Here's how the part is built. I have some questions about the finished solid (model axes, mm). Face numbers are marked on the shaded views. A direction names the side the tool comes from. Give positions to 0.01 mm unless a question says otherwise; leave off trailing zeros. Write each loop counter-clockwise with the first axis right and the second up, starting at its lowest first coordinate (ties: lowest second). Pieces come first, ordered by that corner, then holes. Notation, with made-up numbers: (-29, 17) -> (-20, 17) arc R17 ccw to (-20, 39) -> close; hole circle Ø3 at (75.25, 16.25). An arc over 180 degrees is marked (long way). Use one line per item in the form item = value.
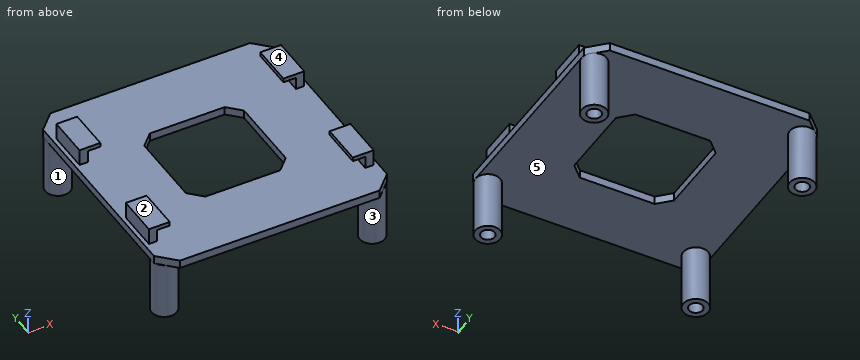
```python
from build123d import *

# Parameters (mm, degrees)
EXTRUDE_START              = -6
EXTRUDE_275_DEPTH          = 2
EXTRUDE_START_2            = -20
SKETCH_2_R                 = 3
EXTRUDE_1_1_DEPTH          = 14
CUT_EXTRUDE_START          = -20
SKETCH_3_R                 = 1.65
CUT_EXTRUDE_M3_1_1_DEPTH   = 14
EXTRUDE_START_3            = -4
SKETCH_4_W                 = 2
SKETCH_4_H                 = 10
EXTRUDE_1_1_2_DEPTH        = 3
EXTRUDE_START_4            = -1
SKETCH_5_W                 = 5
SKETCH_5_H                 = 10
EXTRUDE_1_1_3_DEPTH        = 1
SKETCH_6_R                 = 3
EXTRUDE_1_1_4_DEPTH        = 14
SKETCH_7_R                 = 1.65
CUT_EXTRUDE_M3_1_1_2_DEPTH = 14
SKETCH_8_W                 = 2
SKETCH_8_H                 = 10
EXTRUDE_1_1_5_DEPTH        = 3
SKETCH_9_W                 = 5
SKETCH_9_H                 = 10
EXTRUDE_1_1_6_DEPTH        = 1
SKETCH_10_R                = 3
EXTRUDE_1_1_7_DEPTH        = 14
SKETCH_11_R                = 1.65
CUT_EXTRUDE_M3_1_1_3_DEPTH = 14
SKETCH_12_W                = 2
SKETCH_12_H                = 10
EXTRUDE_1_1_8_DEPTH        = 3
SKETCH_13_W                = 5
SKETCH_13_H                = 10
EXTRUDE_1_1_9_DEPTH        = 1
SKETCH_14_R                = 3
EXTRUDE_1_1_10_DEPTH       = 14
SKETCH_15_R                = 1.65
CUT_EXTRUDE_M3_1_1_4_DEPTH = 14
SKETCH_16_W                = 2
SKETCH_16_H                = 10
EXTRUDE_1_1_11_DEPTH       = 3
SKETCH_17_W                = 5
SKETCH_17_H                = 10
EXTRUDE_1_1_12_DEPTH       = 1


with BuildPart() as part:
    # 草图1 → Extrude 275 (new body)
    with BuildSketch(Plane.XY.offset(EXTRUDE_START)):
        Polygon((-24, -28), (24, -28), (28, -24), (28, 24), (24, 28), (-24, 28), (-28, 24), (-28, -24), align=None)
        Polygon((-9, -12), (9, -12), (12, -9), (12, 9), (9, 12), (-9, 12), (-12, 9), (-12, -9), align=None, mode=Mode.SUBTRACT)
    extrude(amount=EXTRUDE_275_DEPTH)

    # 草图2 → Extrude 1_-1 (add)
    with BuildSketch(Plane.XY.offset(EXTRUDE_START_2)):
        with Locations(Location((-25, -23, 0), (0, 0, 180))):
            Circle(SKETCH_2_R)
    extrude(amount=EXTRUDE_1_1_DEPTH)

    # 草图3 → Cut-Extrude M3__-1_-1 (cut)
    with BuildSketch(Plane.XY.offset(CUT_EXTRUDE_START)):
        with Locations((-25, -23)):
            Circle(SKETCH_3_R)
    extrude(amount=CUT_EXTRUDE_M3_1_1_DEPTH, mode=Mode.SUBTRACT)

    # 草图4 → Extrude 1_-1 2 (add)
    with BuildSketch(Plane.XY.offset(EXTRUDE_START_3)):
        with Locations((-26, -15)):
            Rectangle(SKETCH_4_W, SKETCH_4_H)
    extrude(amount=EXTRUDE_1_1_2_DEPTH)

    # 草图5 → Extrude 1_-1 3 (add)
    with BuildSketch(Plane.XY.offset(EXTRUDE_START_4)):
        with Locations((-24.5, -15)):
            Rectangle(SKETCH_5_W, SKETCH_5_H)
    extrude(amount=EXTRUDE_1_1_3_DEPTH)

    # 草图6 → Extrude 1_1 4 (add)
    with BuildSketch(Plane.XY.offset(EXTRUDE_START_2)):
        with Locations(Location((-25, 23, 0), (0, 0, 180))):
            Circle(SKETCH_6_R)
    extrude(amount=EXTRUDE_1_1_4_DEPTH)

    # 草图7 → Cut-Extrude M3__-1_1 2 (cut)
    with BuildSketch(Plane.XY.offset(CUT_EXTRUDE_START)):
        with Locations((-25, 23)):
            Circle(SKETCH_7_R)
    extrude(amount=CUT_EXTRUDE_M3_1_1_2_DEPTH, mode=Mode.SUBTRACT)

    # 草图8 → Extrude 1_1 5 (add)
    with BuildSketch(Plane.XY.offset(EXTRUDE_START_3)):
        with Locations((-26, 15)):
            Rectangle(SKETCH_8_W, SKETCH_8_H)
    extrude(amount=EXTRUDE_1_1_5_DEPTH)

    # 草图9 → Extrude 1_1 6 (add)
    with BuildSketch(Plane.XY.offset(EXTRUDE_START_4)):
        with Locations((-24.5, 15)):
            Rectangle(SKETCH_9_W, SKETCH_9_H)
    extrude(amount=EXTRUDE_1_1_6_DEPTH)

    # 草图10 → Extrude 1_-1 7 (add)
    with BuildSketch(Plane.XY.offset(EXTRUDE_START_2)):
        with Locations((25, -23)):
            Circle(SKETCH_10_R)
    extrude(amount=EXTRUDE_1_1_7_DEPTH)

    # 草图11 → Cut-Extrude M3__1_-1 3 (cut)
    with BuildSketch(Plane.XY.offset(CUT_EXTRUDE_START)):
        with Locations((25, -23)):
            Circle(SKETCH_11_R)
    extrude(amount=CUT_EXTRUDE_M3_1_1_3_DEPTH, mode=Mode.SUBTRACT)

    # 草图12 → Extrude 1_-1 8 (add)
    with BuildSketch(Plane.XY.offset(EXTRUDE_START_3)):
        with Locations((26, -15)):
            Rectangle(SKETCH_12_W, SKETCH_12_H)
    extrude(amount=EXTRUDE_1_1_8_DEPTH)

    # 草图13 → Extrude 1_-1 9 (add)
    with BuildSketch(Plane.XY.offset(EXTRUDE_START_4)):
        with Locations((24.5, -15)):
            Rectangle(SKETCH_13_W, SKETCH_13_H)
    extrude(amount=EXTRUDE_1_1_9_DEPTH)

    # 草图14 → Extrude 1_1 10 (add)
    with BuildSketch(Plane.XY.offset(EXTRUDE_START_2)):
        with Locations((25, 23)):
            Circle(SKETCH_14_R)
    extrude(amount=EXTRUDE_1_1_10_DEPTH)

    # 草图15 → Cut-Extrude M3__1_1 4 (cut)
    with BuildSketch(Plane.XY.offset(CUT_EXTRUDE_START)):
        with Locations((25, 23)):
            Circle(SKETCH_15_R)
    extrude(amount=CUT_EXTRUDE_M3_1_1_4_DEPTH, mode=Mode.SUBTRACT)

    # 草图16 → Extrude 1_1 11 (add)
    with BuildSketch(Plane.XY.offset(EXTRUDE_START_3)):
        with Locations((26, 15)):
            Rectangle(SKETCH_16_W, SKETCH_16_H)
    extrude(amount=EXTRUDE_1_1_11_DEPTH)

    # 草图17 → Extrude 1_1 12 (add)
    with BuildSketch(Plane.XY.offset(EXTRUDE_START_4)):
        with Locations((24.5, 15)):
            Rectangle(SKETCH_17_W, SKETCH_17_H)
    extrude(amount=EXTRUDE_1_1_12_DEPTH)


solid = part.part
```
Q1. I want a section at B-B, the plane x = -6. Write out the boundary of the cut face in (y, z), and give its area (3 significant figures).
Result set:
outline = (-28, -6) -> (-12, -6) -> (-12, -4) -> (-28, -4) -> close; (12, -6) -> (28, -6) -> (28, -4) -> (12, -4) -> close
area = 64.0 mm2
Q2. I want a section at A-A, the plane z = -9.5. Write out the boundary of the cut face in (x, y), and give its area (3 significant figures).
Result set:
outline = circle Ø6 at (-25, -23); circle Ø6 at (-25, 23); circle Ø6 at (25, -23); circle Ø6 at (25, 23); hole circle Ø3.3 at (-25, -23); hole circle Ø3.3 at (-25, 23); hole circle Ø3.3 at (25, -23); hole circle Ø3.3 at (25, 23)
area = 78.9 mm2
Q3. Will these pins go through, and if not, where does the flat tip stop? pin 1 Ø2 at (x, z) = (24.5, -2.5) entering from +Y; pin 2 Ø1.1 at (y, z) = (-15, -0.5) entering from -X; pin 3 Ø1.5 at (y, z) = (-14.5, -2.5) entering from +X; pin 4 Ø3 at (x, z) = (-20, -15.5) entering from +Y.
Result set:
pin_1 = 20
pin_2 = -27
pin_3 = 27
pin_4 = through
Q4. If we mould it in two halves opening along Y, with no side actions, what happens to the marked faces 3, 4 and 5? For each: +Y half, -Y half, draft (parallel to the pull), parting line (faces both ways), or undercut.
Result set:
face_3 = undercut
face_4 = draft
face_5 = undercut
Q5. I want a section at C-C, the plane z = -3. Write out the boundary of the cut face in (x, y), and give its area (3 significant figures).
Result set:
outline = (-27, -20) -> (-25, -20) -> (-25, -10) -> (-27, -10) -> close; (-27, 10) -> (-25, 10) -> (-25, 20) -> (-27, 20) -> close; (25, -20) -> (27, -20) -> (27, -10) -> (25, -10) -> close; (25, 10) -> (27, 10) -> (27, 20) -> (25, 20) -> close
area = 80.0 mm2
Q6. Which directions (+Z, -Z, +X, -X, +Y, -Y) give clear straight access to the entire face, cutting with the end or side of a thin tool? Please do the marked faces 1 and 2.
Result set:
face_1 = -Z
face_2 = +Z, +X, -X, +Y, -Y
Q7. If I drill on line 1 along Y through (x, z) = (-25, -9.75); line 2 along Y through (x, z) = (5, -4.25), over which ranges is the centre line in solid material (lowest first)? Write a range as from..to.
Result set:
line_1 = -26..-24.65, -21.35..-20, 20..21.35, 24.65..26
line_2 = -28..-12, 12..28
